Read the model definition and answer for the solid it produces. Units are mm, in the model's axes. A direction names the side the tool comes from. Round coordinates to 2 decimals unless told otherwise and drop trailing zeros. Write each loop counter-clockwise with the first axis right and the second up, starting at its lowest first coordinate (ties: lowest second). Pieces come first, ordered by that corner, then holes. Notation, with made-up numbers: (60.5, 15) -> (95.5, 15) arc R20 ccw to (95.5, 48) -> close; hole circle Ø9 at (76, -2.75). An arc over 180 degrees is marked (long way). Return JSON: item names as keys, results as strings. Group by question number.
(1) For faces 1 (the flat face through (-11, -11, -12.7)), 2 (the cylindrical face through (2.75, 12.4, -272.96)), 3 (the flat face through (0, 0, 0)), determine the directions among +Z, -Z, +X, -X, +Y, -Y from which every point of the face is accessible in a straight line to the end or side of a thin tool.
(2) Straight lines are drawn through the part: line 1 (Z direction, x = 26, y = -8); line 2 (X direction, y = -2, z = -161.5); line 3 (X direction, y = -25, z = -15). For each, find the intervals that lie inside material, in ascending order.
(3) Given pin 1 (3 mm diameter, centred on y = 10.5, z = -162.5, fed in from -X); pin 2 (3 mm diameter, centred on y = -34, z = -193.5, fed in from +X); pin 3 (3 mm diameter, centred on y = -16, z = -49.5, fed in from -X), each flat-ended and moving along its own axis, determine where each tip first touches the part or whether it passes through.
(4) A cutting plane is placed at D-D on y = -27. Give the vertices of the cut face in (x, z).
(5) A cutting plane is placed at C-C on z = -217. Give the vertices of the cut face in (x, y).
(6) A cutting plane is placed at A-A on y = 0. Give the vertices of the cut face in (x, z).
Autodesk Inventor part; units mm, degrees
ref_plane "YZ Plane" through (0, 0, 0) normal (1, 0, 0) x (0, 1, 0)
ref_plane "XZ Plane" through (0, 0, 0) normal (0, 1, 0) x (-1, 0, 0)
ref_plane "XY Plane" through (0, 0, 0) normal (0, 0, 1) x (1, 0, 0)
sketch "Sketch1" plane through (0, 0, 0) normal (0, 0, 1) x (1, 0, 0)
  circle A0 centre (0, 0) radius 31.75
  dimension "d0" = 63.5
extrude "Extrusion1" add sketch "Sketch1" along normal blind 82.55
sketch "Sketch2" plane through (0, 0, 82.55) normal (0, 0, 1) x (1, 0, 0)
  circle A0 centre (0, 0) radius 31.75
  circle A1 centre (0, 0) radius 14.859
  dimension "d3" = 29.718
extrude "Extrusion2" add sketch "Sketch2" along normal blind 6.35 contours A1
sketch "Sketch3" plane through (0, 0, 0) normal (0, 0, -1) x (-1, 0, 0)
  circle A0 centre (0, 0) radius 31.75
  circle A1 centre (0, 0) radius 12.7
  dimension "d6" = 25.4
extrude "Extrusion3" add sketch "Sketch3" along normal blind 12.7 contours A1
sketch "Sketch4" plane through (0, 0, -12.7) normal (0, 0, -1) x (-1, 0, 0)
  circle A0 centre (0, 0) radius 12.7
  circle A1 centre (0, 0) radius 50.8
  dimension "d9" = 101.6
extrude "Extrusion4" add sketch "Sketch4" along normal blind 254 contours A0 | A1
sketch "Sketch5" plane through (0, 0, -266.7) normal (0, 0, -1) x (-1, 0, 0)
  circle A0 centre (0, 0) radius 50.8
  circle A1 centre (0, 0) radius 12.7
  dimension "d12" = 25.4
extrude "Extrusion5" add sketch "Sketch5" along normal blind 12.7 contours A1
sketch "Sketch7" plane through (0, 0, 88.9) normal (0, 0, 1) x (1, 0, 0)
  circle A0 centre (0, 0) radius 14.859
  circle A1 centre (0, 0) radius 117.3057
extrude "Extrusion6" cut sketch "Sketch7" against normal blind 88.9 contours A0 | A1
properties part number "Shooter_RollerTop"
Checks:
{
 "1": {"face 1": "+Z", "face 2": "-Z", "face 3": "+Z, +X, -X, +Y, -Y"},
 "2": {"line 1": "z = -266.7 to -12.7", "line 2": "x = -50.76 to 50.76", "line 3": "x = -44.22 to 44.22"},
 "3": {"pin 1": "stops at x = -50", "pin 2": "stops at x = 39.04", "pin 3": "stops at x = -48.69"},
 "4": {"outline": "(-43.03, -266.7) -> (43.03, -266.7) -> (43.03, -12.7) -> (-43.03, -12.7) -> close"},
 "5": {"outline": "circle Ø101.6 at (0, 0)"},
 "6": {"outline": "(-50.8, -266.7) -> (-12.7, -266.7) -> (-12.7, -279.4) -> (12.7, -279.4) -> (12.7, -266.7) -> (50.8, -266.7) -> (50.8, -12.7) -> (12.7, -12.7) -> (12.7, 0) -> (-12.7, 0) -> (-12.7, -12.7) -> (-50.8, -12.7) -> close"}
}
